Autodesk Inventor part; units mm, degrees
ref_plane "YZ Plane" through (0, 0, 0) normal (1, 0, 0) x (0, 1, 0)
ref_plane "XZ Plane" through (0, 0, 0) normal (0, 1, 0) x (-1, 0, 0)
ref_plane "XY Plane" through (0, 0, 0) normal (0, 0, 1) x (1, 0, 0)
sketch "Sketch3" plane through (0, 0, 0) normal (0, 0, 1) x (1, 0, 0)
  circle A0 centre (0, 0) radius 11.5
  circle A1 centre (0, 0) radius 3
  circle A2 centre (7, 0) radius 1.5
  circle A3 centre (3.5, 6.0622) radius 1.5
  circle A4 centre (-3.5, 6.0622) radius 1.5
  circle A5 centre (-7, 0) radius 1.5
  circle A6 centre (-3.5, -6.0622) radius 1.5
  circle A7 centre (3.5, -6.0622) radius 1.5
  dimension "d0" = 23
  dimension "d1" = 6
  dimension "d4" = 3
  dimension "d5" = 7
  dimension "d12" = 360
extrude "Extrusion1" add sketch "Sketch3" along normal blind 5 contours A0 | A3 | A5 | A7
sketch "Sketch4" plane through (0, 0, 0) normal (1, 0, 0) x (0, 1, 0)
  line L0 (-11.5, 0) -> (11.5, 0)
  line L1 (-3, 5) -> (3, 5)
  line L2 (3, 0) -> (-3, 0)
  circle A0 centre (0, 2.5) radius 1.5
  line L3 (3, 0) -> (3, 5)
  point P0 (0, 0)
  point P1 (0, 0)
  point P2 (3, 2.5)
  dimension "d14" = 3
extrude "Extrusion2" cut sketch "Sketch4" against normal through all
thread "Thread1"
thread "Thread2"
thread "Thread3"
thread "Thread4"
sketch "Sketch5" plane through (0, 0, 5) normal (0, 0, 1) x (1, 0, 0)
  line L0 (3.7445, 8.0908) -> (6.8872, 8.0908)
  line L1 (6.8872, 8.0908) -> (6.8872, 3.8114)
  line L2 (6.8872, 3.8114) -> (3.7445, 3.8114)
  line L3 (3.7445, 3.8114) -> (3.7445, 8.0908)
  point P0 (0, 0)
extrude "Extrusion3" cut sketch "Sketch5" against normal blind 0.1
equation "\"d15\" = d14"
properties part number "6mm Mounting Hub, thin" material "Aluminum 6061"
The model under review builds one solid part; all positions refer to its coordinate system, in mm. A direction names the side the tool comes from. Round coordinates to 2 decimals unless told otherwise and drop trailing zeros. Write each loop counter-clockwise with the first axis right and the second up, starting at its lowest first coordinate (ties: lowest second). Pieces come first, ordered by that corner, then holes. Notation, with made-up numbers: M -14,49.25 L -1,49.25 A23 ccw -1,63.25 Z; hole C 31,-36 d1. An arc over 180 degrees is marked long. Use a Markdown table: item, result. Add a question column.
Q1. We need section B-B, the plane y = 5. State the section outline as (x, z) points, plus the area to 3 significant figures.
Q2. We need section A-A, the plane x = -3.5. State the section outline as (y, z) points.
Q3. We need section C-C, the plane z = 3.2. State the section outline as (x, y) points.
Q4. Machinability: for faces 1 (the face through (5.5, -0.07, 2.46)), 2 (the face through (5, 6, 4.9)), which of the approach directions +Z, -Z, +X, -X, +Y, -Y give a long, thin tool a straight path to every point of the face, cutting with its end or side? Answer none if there is none.
Q5. To check wall thickness, follow line 1 (Y direction, x = -3.5, z = 1.6); line 2 (X direction, y = -0.75, z = 0.35); line 3 (X direction, y = 7, z = 0.7). State the ranges of each line that lie inside material, in increasing order.
Q6. Insertion check: pin 1 (2 mm diameter, centred on y = 2, z = 3, fed in from -X); pin 2 (10 mm diameter, centred on x = -4, y = -3.5, fed in from -Z); pin 3 (3 mm diameter, centred on y = -5, z = 4, fed in from -X); pin 4 (0.9 mm diameter, centred on x = 6, y = 7, fed in from +Z). Each pin has a flat end and moves straight along its axis. Give the tip position at first contact, or say it passes through.
Q7. We need section D-D, the plane x = 0. State the section outline as (y, z) points.
Q8. The part is to be moulded in two halves that separate along Z. For faces 3 (the face through (-2.1, 6.6, 2.5)), 4 (the face through (-7, 0, 1)), 5 (the face through (2.4, -2.4, 0)), say which applies: pulls with the +Z half, pulls with the -Z half, needs draft (parallel to the pull), parting line crosses it, or undercut.
Findings below:
| question | item | result |
|---|---|---|
| 1 | outline | M -10.36,0 L -4.56,0 L -4.56,5 L -10.36,5 Z; M -2.44,0 L 10.36,0 L 10.36,5 L 6.89,5 L 6.89,4.9 L 3.74,4.9 L 3.74,5 L -2.44,5 Z |
| 1 | area | 92.7 mm² |
| 2 | outline | M -10.95,0 L -7.56,0 L -7.56,5 L -10.95,5 Z; M -4.56,0 L 4.56,0 L 4.56,5 L -4.56,5 Z; M 7.56,0 L 10.95,0 L 10.95,5 L 7.56,5 Z; hole C 0,2.5 d3 |
| 3 | outline | M -11.42,-1.33 A11.5 ccw long -11.42,1.33 L -2.69,1.33 A3 cw long -2.69,-1.33 Z; hole C -3.5,-6.06 d3; hole C -3.5,6.06 d3; hole C 7,0 d3 |
| 4 | face 1 | +Z, -Z |
| 4 | face 2 | +Z |
| 5 | line 1 | y = -10.95 to -7.56, -4.56 to -1.2, 1.2 to 4.56, 7.56 to 10.95 |
| 5 | line 2 | x = -11.48 to -2.9, 2.9 to 5.7, 8.3 to 11.48 |
| 5 | line 3 | x = -9.12 to -4.67, -2.33 to 9.12 |
| 6 | pin 1 | stops at x = -11.44 |
| 6 | pin 2 | stops at z = 0 |
| 6 | pin 3 | stops at x = -10.95 |
| 6 | pin 4 | stops at z = 4.9 |
| 7 | outline | M -11.5,0 L -3,0 L -3,5 L -11.5,5 Z; M 3,0 L 11.5,0 L 11.5,5 L 3,5 Z |
| 8 | face 3 | needs draft |
| 8 | face 4 | undercut |
| 8 | face 5 | pulls with the -Z half |
